Work out the finished part from the listing and answer in its coordinate system (mm). A direction names the side the tool comes from. Give positions to 0.01 mm unless a question says otherwise; leave off trailing zeros. Order: outer loops, then holes, each group sorted by start corner. A loop starts at its lowest first (then second) coordinate and runs counter-clockwise, first axis right, second up. Notation, with made-up numbers: (87, 71.25) -> (118, 71.25) arc R12 cw to (118, 80.25) -> close; hole circle Ø4 at (1, 37.5). An arc over 180 degrees is marked (long way). Answer as CSV lines item,"result". Start each with the question number.
1. For a pull along Y with two mould halves and no side action, classify faces 1 (the flat face through (10, -30, 14)), 2 (the cylindrical face through (-113.97, -231.534, 4.303)), 3 (the cylindrical face through (75.874, -254.216, 14.67)) as released by +Y, released by -Y, zero draft, split by the parting line, or undercut.
2. A cutting plane is placed at A-A (y = -170). Give the vertices of the cut face in (x, z).
3. A cutting plane is placed at D-D (y = -85.5). Give the vertices of the cut face in (x, z).
4. For faces 4 (the flat face through (-10, -30, 14)), 5 (the flat face through (-122, -240, 8.727)), 6 (the flat face through (114, -253, 18.727)), determine the directions among +Z, -Z, +X, -X, +Y, -Y from which every point of the face is accessible in a straight line to the end or side of a thin tool.
5. Flat-ended cylindrical pins translate along their axes: pin 1 (1.5 mm diameter, centred on x = 110, z = 3.5, fed in from -Y); pin 2 (1.5 mm diameter, centred on y = -146.5, z = 4.5, fed in from -X); pin 3 (10 mm diameter, centred on y = -36.5, z = 13.5, fed in from +X). Find the tip coordinate at first contact, or state that the pin passes through.
6. A cutting plane is placed at B-B (x = -24.5). Give the vertices of the cut face in (y, z), then the cut area to 3 significant figures.
7. A cutting plane is placed at C-C (y = -14). Give the vertices of the cut face in (x, z), then the cut area to 3 significant figures.
8. Find the intervals of material crossed by L1, parallel to Y at x = 0.5, z = 14.5; L2, parallel to X at y = -39, z = 2; L3, parallel to X at y = -248, z = 12.5, in increasing order.
from build123d import *

# Parameters (mm, degrees)
F1_DEPTH  = 60
F3_DEPTH  = 5
F4_R      = 4
F5_DEPTH  = 30.001
F6_DEPTH  = 10
F10_COUNT = 3
F10_ANGLE = 240
F8_W      = 110
F8_H      = 30
F12_R     = 100
F13_DEPTH = 20
F14_R     = 17.5157850189
F15_DEPTH = 10.0010001


with BuildPart() as f1:
    # F0 (on Front) → F1 (new body)
    with BuildSketch(Plane.XZ):
        Polygon((-20, 18.7272732889), (-20, 0), (20, 0), (20, 18.7272732889), (10, 18.7272732889), (10, 8.7272732889), (-10, 8.7272732889), (-10, 18.7272732889), align=None)
    extrude(amount=F1_DEPTH)

    # F2 (on face) → F3 (join)
    with BuildSketch(Plane.XZ.offset(60)):
        with BuildLine():
            ThreePointArc((-20, 30), (-35, 15), (-20, 0))
            Line((-20, 0), (20, 0))
            ThreePointArc((20, 0), (35, 15), (20, 30))
            Line((20, 30), (-20, 30))
        make_face()
    extrude(amount=F3_DEPTH)

    # F4 (on Top) → F5 (cut, through all)
    with BuildSketch(Plane.XY):
        with Locations((0, -39)):
            Circle(F4_R)
        with Locations((0, -14)):
            Circle(F4_R)
    extrude(amount=F5_DEPTH, mode=Mode.SUBTRACT)

    # F2 (on face) → F6 (join)
    with BuildSketch(Plane.XZ.offset(60)):
        with BuildLine():
            ThreePointArc((-20, 30), (-35, 15), (-20, 0))
            Line((-20, 0), (20, 0))
            ThreePointArc((20, 0), (35, 15), (20, 30))
            Line((20, 30), (-20, 30))
        make_face()
    extrude(amount=F6_DEPTH)


with BuildPart() as f10_1:
    # F10: instance of F1
    add(f1.part.rotate(Axis((0, -170, 15), (0, 0, 1)), 1 * F10_ANGLE / (F10_COUNT - 1)))


with BuildPart() as f10_2:
    # F10: instance of F1
    add(f1.part.rotate(Axis((0, -170, 15), (0, 0, 1)), 2 * F10_ANGLE / (F10_COUNT - 1)))


with BuildPart() as f1_1:
    add(f1.part)

    add(f10_1.part)  # F11 merges F10_1

    add(f10_2.part)  # F11 merges F10_2
    # F8 (on offset) → F11 (revolve)
    with BuildSketch(Plane.XZ.offset(170)):
        with Locations((55, 15)):
            Rectangle(F8_W, F8_H)
    revolve(axis=Axis((0, -170, 4.4428613037), (0, 0, 1)))

    # F12 (on face) → F13 (cut)
    with BuildSketch(Plane.XY.offset(30)):
        with Locations((0, -170)):
            Circle(F12_R)
    extrude(amount=-F13_DEPTH, mode=Mode.SUBTRACT)

    # F14 (on face) → F15 (cut, through all)
    with BuildSketch(Plane.XY.offset(10)):
        with Locations((0, -170)):
            Circle(F14_R)
    extrude(amount=-F15_DEPTH, mode=Mode.SUBTRACT)


solid = f1_1.part
Answer sheet:
1,face 1,"zero draft"
1,face 2,"undercut"
1,face 3,"released by -Y"
2,outline,"(-110, 0) -> (-17.52, 0) -> (-17.52, 10) -> (-100, 10) -> (-100, 30) -> (-110, 30) -> close; (17.52, 0) -> (110, 0) -> (110, 30) -> (100, 30) -> (100, 10) -> (17.52, 10) -> close"
3,outline,"(-70.43, 0) -> (70.43, 0) -> (70.43, 30) -> (53.48, 30) -> (53.48, 10) -> (-53.48, 10) -> (-53.48, 30) -> (-70.43, 30) -> close"
4,face 4,"+Z, +Y"
4,face 5,"+Z"
4,face 6,"+Z, +X, -Y"
5,pin 1,"stops at y = -257.04"
5,pin 2,"stops at x = -107.62"
5,pin 3,"stops at x = 20"
6,outline,"(-277.24, 0) -> (-62.76, 0) -> (-62.76, 0.69) -> (-60, 0.69) -> (-60, 29.31) -> (-62.76, 29.31) -> (-62.76, 30) -> (-73.05, 30) -> (-73.05, 10) -> (-266.95, 10) -> (-266.95, 30) -> (-277.24, 30) -> close"
6,area,"2,640 mm^2"
7,outline,"(-20, 0) -> (-4, 0) -> (-4, 8.73) -> (-10, 8.73) -> (-10, 18.73) -> (-20, 18.73) -> close; (4, 0) -> (20, 0) -> (20, 18.73) -> (10, 18.73) -> (10, 8.73) -> (4, 8.73) -> close"
7,area,"479 mm^2"
8,L1,"y = -280 to -270, -70 to -60"
8,L2,"x = -20 to -4, 4 to 20"
8,L3,"x = -115.1 to -95.1, -81.98 to -62.58, 62.58 to 81.98, 95.1 to 115.1"
